from build123d import *

# Parameters (mm, degrees)
BOSS_EXTRUDE3_DEPTH = 5
SKETCH32_W          = 10
SKETCH32_H          = 10
BOSS_EXTRUDE5_DEPTH = 57.810843841
SKETCH33_W          = 30
SKETCH33_H          = 30
BOSS_EXTRUDE6_DEPTH = 10
FILLET2_R           = 5
SKETCH34_R          = 2
CUT_EXTRUDE2_DEPTH  = 4


with BuildPart() as part:
    # Sketch11 → Boss-Extrude3 (new, symmetric)
    with BuildSketch(Plane.XY):
        Polygon((-70, 130), (-70, 117.810843841), (0, 53.195459226), (70, 117.810843841), (70, 130), (60, 130), (60, 122.189156159), (0, 66.804540774), (-60, 122.189156159), (-60, 130), align=None)
    extrude(amount=BOSS_EXTRUDE3_DEPTH, both=True)

    # Sketch32 → Boss-Extrude5 (add)
    with BuildSketch(Plane(origin=(0, 0, 0), x_dir=(1, 0, 0), z_dir=(0, 1, 0))):
        Rectangle(SKETCH32_W, SKETCH32_H)
    extrude(amount=BOSS_EXTRUDE5_DEPTH)

    # Sketch33 → Boss-Extrude6 (add)
    with BuildSketch(Plane.XZ):
        Rectangle(SKETCH33_W, SKETCH33_H)
    extrude(amount=-BOSS_EXTRUDE6_DEPTH)

    # Fillet2
    fillet2_edges = [part.edges().sort_by_distance(p)[0] for p in [
        (-5, 10, 0),
        (0, 10, -5),
        (15, 10, 0),
        (0, 10, -15),
        (-15, 10, 0),
        (0, 10, 15),
        (0, 10, 5),
        (5, 10, 0),
    ]]
    fillet(fillet2_edges, radius=FILLET2_R - 0.0001)  # a hair under: the kernel refuses the full size

    # Sketch34 → Cut-Extrude2 (cut)
    with BuildSketch(Plane(origin=(0, 130, 0), x_dir=(1, 0, 0), z_dir=(0, 1, 0))):
        with Locations(Location((-65, 0, 0), (0, 0, 270))):
            Circle(SKETCH34_R)
        with Locations(Location((65, 0, 0), (0, 0, 270))):
            Circle(SKETCH34_R)
    extrude(amount=-CUT_EXTRUDE2_DEPTH, mode=Mode.SUBTRACT)


solid = part.part
Model file for the job. Use its own axes, mm. A direction names the side the tool comes from. Give positions to 0.01 mm unless a question says otherwise; leave off trailing zeros. Order: outer loops, then holes, each group sorted by start corner. A loop starts at its lowest first (then second) coordinate and runs counter-clockwise, first axis right, second up. Notation, with made-up numbers: (19, 0.25) - (33, 0.25) arc R18 cw to (33, 12.25) - close; hole circle Ø6 at (61.5, 26.5). An arc over 180 degrees is marked (long way). One line per item, written item: value.
Item 1: Two-plate mould, pull along Z, no slides. Class faces 1 (the flat face through (-62.7, 130, 0.1)), 2 (the cylindrical face through (-63, 128, 0)), 3 (the flat face through (-65, 126, 0)), 4 (the cylindrical face through (0, 11, 7)): released by +Z, released by -Z, zero draft, split by the parting line, or undercut.
Response values:
face 1: zero draft
face 2: undercut
face 3: undercut
face 4: released by +Z
Item 2: Slice it at B-B (x = -65). List the corners of the cut face in (y, z), then the cut area to 3 significant figures.
Response values:
outline: (113.2, -5) - (130, -5) - (130, -2) - (126, -2) - (126, 2) - (130, 2) - (130, 5) - (113.2, 5) - close
area: 152 mm2
Item 3: Pin check, flat tips, straight feed: pin 1 Ø10 at (y, z) = (29.5, 4) entering from +X; pin 2 Ø3 at (x, z) = (65.5, 1) entering from +Y; pin 3 Ø4 at (y, z) = (1.5, -6.5) entering from -X; pin 4 Ø2.5 at (y, z) = (1.5, -3) entering from +X. Stop position of each tip, or through.
Response values:
pin 1: x = 5
pin 2: y = 130
pin 3: x = -15
pin 4: x = 15
Item 4: Wall check: line 1 (X direction, y = 129, z = 0); line 2 (Y direction, x = -7.5, z = -0.75); line 3 (Y direction, x = 4.5, z = -10.25). Give the ranges that are in metal, low to high.
Response values:
line 1: -70 to -67, -63 to -60, 60 to 63, 67 to 70
line 2: 0 to 10.67, 60.12 to 73.73
line 3: 0 to 9.99
Item 5: Slice it at C-C (z = -12.75). List the corners of the cut face in (x, y), then the cut area to 3 significant figures.
Response values:
outline: (-15, 0) - (15, 0) - (15, 5) arc R5 ccw to (12.75, 9.18) - (-12.75, 9.18) arc R5 ccw to (-15, 5) - close
area: 270 mm2
Item 6: Slice it at D-D (y = 44). List the corners of the cut face in (x, z), then the cut area to 3 significant figures.
Response values:
outline: (-5, -5) - (5, -5) - (5, 5) - (-5, 5) - close
area: 100 mm2
Item 7: Tool access for faces 5 (the cylindrical face through (66.686, 128.028, 1.075)), 6 (the cylindrical face through (13, 9, 0)), 7 (the flat face through (30.42, 94.885, 0.07)): list every direction of +Z, -Z, +X, -X, +Y, -Y with a clear straight run to the whole face (end or side of a thin tool).
Response values:
face 5: +Y
face 6: +Z, -Z, +X
face 7: +Z, -Z, +Y
Item 8: Slice it at A-A (y = 114.5). List the corners of the cut face in (x, z).
Response values:
outline: (-66.41, -5) - (-51.67, -5) - (-51.67, 5) - (-66.41, 5) - close; (51.67, -5) - (66.41, -5) - (66.41, 5) - (51.67, 5) - close
